The listing builds one solid part. Answer for the finished solid, in the listing's coordinates (mm). A direction names the side the tool comes from. Give positions to 0.01 mm unless a question says otherwise; leave off trailing zeros. Loops run counter-clockwise (first coordinate to the right, second up) from the corner with the lowest first, then second, coordinate; pieces in that order, holes last. Notation, with made-up numbers: M -31,-38 L -25,-38 A29 cw -25,-16 Z; hole C 36,85 d7. An arc over 180 degrees is marked long. One line per item, written item: value. Start each with the question number.
Q1. For faces 1 (the flat face through (9.3, 5, 0.9)), 2 (the flat face through (0, 4.9, 0.5)), 3 (the flat face through (19.653, 8.115, 0.507)), determine the directions among +Z, -Z, +X, -X, +Y, -Y from which every point of the face is accessible in a straight line to the end or side of a thin tool.
Q2. The mould has two halves that part along Y. Classify faces 4 (the cylindrical face through (21.4, 5, 0.5)), 5 (the cylindrical face through (18.6, 5, 0.5)), 6 (the flat face through (9.5, 5.1, 0)), 7 (the flat face through (12.3, 10, 0.5)): +Y half, -Y half, draft (parallel to the pull), parting line (faces both ways), or undercut.
Q3. A cutting plane is placed at A-A, the plane x = 5. Determine the outline of the cut face in (y, z).
Q4. A cutting plane is placed at D-D, the plane x = 12. Determine the outline of the cut face in (y, z), and give its area (3 significant figures).
Q5. A cutting plane is placed at B-B, the plane y = 5. Determine the outline of the cut face in (x, z), and give its area (3 significant figures).
Q6. A cutting plane is placed at C-C, the plane z = 0.75. Determine the outline of the cut face in (x, y), and give its area (3 significant figures).
Q7. Consider L1, parallel to X at y = 5, z = 0.85; L2, parallel to Y at x = 11.5, z = 0.85; L3, parallel to Y at x = 5, z = 0.75. Determine where each line is inside the solid, lowest interval first.
from build123d import *

# Parameters (mm, degrees)
CYLINDER002_W               = 13.6
CYLINDER002_H               = 11
CYLINDER002_ANGLE           = 24
CYLINDER002_PLACEMENT_ANGLE = -12
CYLINDER001_W               = 16.4
CYLINDER001_H               = 10
CYLINDER001_ANGLE           = 24
CYLINDER001_PLACEMENT_ANGLE = -12
CYLINDER_R                  = 1.3
CYLINDER_DEPTH              = 10
BOX002_W                    = 7
BOX002_H                    = 7
BOX002_DEPTH                = 0.5
BOX001_W                    = 5
BOX001_H                    = 5
BOX001_DEPTH                = 2
BOX_W                       = 25
BOX_H                       = 10
BOX_DEPTH                   = 1


with BuildPart() as zylinder002:
    # Cylinder002 → Cylinder002 (revolve)
    with BuildSketch(Plane.XZ):
        with Locations((6.8, 5.5)):
            Rectangle(CYLINDER002_W, CYLINDER002_H)
    revolve(axis=Axis((0, 0, 0), (0, 0, 1)), revolution_arc=CYLINDER002_ANGLE)


with BuildPart() as zylinder002_1:
    # Cylinder002 placement: moved
    add(zylinder002.part.moved(Location((3, 5, 0))).rotate(Axis((3, 5, 0), (0, 0, 1)), CYLINDER002_PLACEMENT_ANGLE))


with BuildPart() as cut:
    # Cylinder001 → Cylinder001 (revolve)
    with BuildSketch(Plane.XZ):
        with Locations((8.2, 5)):
            Rectangle(CYLINDER001_W, CYLINDER001_H)
    revolve(axis=Axis((0, 0, 0), (0, 0, 1)), revolution_arc=CYLINDER001_ANGLE)


with BuildPart() as cut_1:
    # Cylinder001 placement: moved
    add(cut.part.moved(Location((3, 5, 0))).rotate(Axis((3, 5, 0), (0, 0, 1)), CYLINDER001_PLACEMENT_ANGLE))

    # Cut: cut Zylinder002
    add(zylinder002_1.part, mode=Mode.SUBTRACT)


with BuildPart() as cut_2:
    # Cut placement: moved
    add(cut_1.part.moved(Location((2, 0, 0))))


with BuildPart() as zylinder:
    # Cylinder → Cylinder (new body)
    with BuildSketch(Plane(origin=(5, 5, 0), x_dir=(1, 0, 0), z_dir=(0, 0, 1))):
        Circle(CYLINDER_R)
    extrude(amount=CYLINDER_DEPTH)


with BuildPart() as obj1:
    # Box002 → Box002 (new body)
    with BuildSketch(Plane(origin=(9, 1.5, 0.9), x_dir=(1, 0, 0), z_dir=(0, 0, 1))):
        with Locations((3.5, 3.5)):
            Rectangle(BOX002_W, BOX002_H)
    extrude(amount=BOX002_DEPTH)


with BuildPart() as obj2:
    # Box001 → Box001 (new body)
    with BuildSketch(Plane(origin=(10, 2.5, 0), x_dir=(1, 0, 0), z_dir=(0, 0, 1))):
        with Locations((2.5, 2.5)):
            Rectangle(BOX001_W, BOX001_H)
    extrude(amount=BOX001_DEPTH)


with BuildPart() as cut004:
    # Box → Box (new body)
    with BuildSketch(Plane.XY):
        with Locations((12.5, 5)):
            Rectangle(BOX_W, BOX_H)
    extrude(amount=BOX_DEPTH)

    # Cut001: cut obj2
    add(obj2.part, mode=Mode.SUBTRACT)

    # Cut002: cut obj1
    add(obj1.part, mode=Mode.SUBTRACT)

    # Cut003: cut Zylinder
    add(zylinder.part, mode=Mode.SUBTRACT)

    # Cut004: cut Cut
    add(cut_2.part, mode=Mode.SUBTRACT)


solid = cut004.part
Answer block:
1. face 1: +Z
1. face 2: +Z, -Z, -X, +Y, -Y
1. face 3: +Z, -Z
2. face 4: undercut
2. face 5: undercut
2. face 6: draft
2. face 7: +Y half
3. outline: M 0,0 L 3.7,0 L 3.7,1 L 0,1 Z; M 6.3,0 L 10,0 L 10,1 L 6.3,1 Z
4. outline: M 0,0 L 2.5,0 L 2.5,0.9 L 1.5,0.9 L 1.5,1 L 0,1 Z; M 7.5,0 L 10,0 L 10,1 L 8.5,1 L 8.5,0.9 L 7.5,0.9 Z
4. area: 4.80 mm^2
5. outline: M 0,0 L 3.7,0 L 3.7,1 L 0,1 Z; M 6.3,0 L 10,0 L 10,0.9 L 9,0.9 L 9,1 L 6.3,1 Z; M 15,0 L 18.6,0 L 18.6,1 L 16,1 L 16,0.9 L 15,0.9 Z; M 21.4,0 L 25,0 L 25,1 L 21.4,1 Z
5. area: 14.4 mm^2
6. outline: M 0,0 L 25,0 L 25,10 L 0,10 Z; hole C 5,5 d2.6; hole M 10,2.5 L 15,2.5 L 15,7.5 L 10,7.5 Z; hole M 18.3,2.17 L 21.04,1.59 A16.4 ccw 21.04,8.41 L 18.3,7.83 A13.6 cw Z
6. area: 202 mm^2
7. L1: 0 to 3.7, 6.3 to 10, 15 to 18.6, 21.4 to 25
7. L2: 0 to 2.5, 7.5 to 10
7. L3: 0 to 3.7, 6.3 to 10
